Read the model definition and answer for the solid it produces. Units are mm, in the model's axes. A direction names the side the tool comes from. Give positions to 0.01 mm unless a question says otherwise; leave off trailing zeros. Order: outer loops, then holes, each group sorted by start corner. A loop starts at its lowest first (then second) coordinate and runs counter-clockwise, first axis right, second up. Notation, with made-up numbers: (76, 44.5) - (86, 44.5) arc R12 cw to (86, 61.5) - close; hole circle Ø6 at (11, 42). An arc over 180 degrees is marked (long way). One line per item, written item: value. Start each with the question number.
```python
from build123d import *

# Parameters (mm, degrees)
BOSS_EXTRU_1_DEPTH      = 3
ESQUISSE2_R             = 1.5
ENL_V_MAT_EXTRU_2_DEPTH = 3
ESQUISSE3_R             = 6
ESQUISSE3_R_2           = 1.5
ENL_V_MAT_EXTRU_3_DEPTH = 10


with BuildPart() as part:
    # Esquisse1 → Boss.-Extru.1 (new body)
    with BuildSketch(Plane.XY):
        Polygon((-50, -75), (50, -75), (50, -65), (60, -65), (60, 75), (-60, 75), (-60, -65), (-50, -65), align=None)
        with BuildLine():
            ThreePointArc((-41.5, 22), (-43, 20.5), (-44.5, 22))
            Line((-44.5, 22), (-44.5, 37))
            ThreePointArc((-44.5, 37), (-43, 38.5), (-41.5, 37))
            Line((-41.5, 37), (-41.5, 22))
        make_face(mode=Mode.SUBTRACT)
        with BuildLine():
            Line((-10.5, 37), (-10.5, 22))
            ThreePointArc((-10.5, 22), (-12, 20.5), (-13.5, 22))
            Line((-13.5, 22), (-13.5, 37))
            ThreePointArc((-13.5, 37), (-12, 38.5), (-10.5, 37))
        make_face(mode=Mode.SUBTRACT)
        with BuildLine():
            ThreePointArc((-41.5, 53), (-43, 51.5), (-44.5, 53))
            Line((-44.5, 53), (-44.5, 68))
            ThreePointArc((-44.5, 68), (-43, 69.5), (-41.5, 68))
            Line((-41.5, 68), (-41.5, 53))
        make_face(mode=Mode.SUBTRACT)
        with BuildLine():
            ThreePointArc((-16.25, 37.5), (-27.5, 26.25), (-38.75, 37.5))
            Line((-38.75, 37.5), (-38.75, 52.5))
            ThreePointArc((-38.75, 52.5), (-27.5, 63.75), (-16.25, 52.5))
            Line((-16.25, 52.5), (-16.25, 37.5))
        make_face(mode=Mode.SUBTRACT)
        with BuildLine():
            Line((-10.5, 68), (-10.5, 53))
            ThreePointArc((-10.5, 53), (-12, 51.5), (-13.5, 53))
            Line((-13.5, 53), (-13.5, 68))
            ThreePointArc((-13.5, 68), (-12, 69.5), (-10.5, 68))
        make_face(mode=Mode.SUBTRACT)
    extrude(amount=BOSS_EXTRU_1_DEPTH)

    # Esquisse2 → Enlèv. mat.-Extru.2 (cut)
    with BuildSketch(Plane.XY.offset(3)):
        with Locations((45, -70)):
            Circle(ESQUISSE2_R)
        with Locations((-55, -60)):
            Circle(ESQUISSE2_R)
        with Locations((-55, 5)):
            Circle(ESQUISSE2_R)
        with Locations((-55, 70)):
            Circle(ESQUISSE2_R)
        with Locations((22.5, -70)):
            Circle(ESQUISSE2_R)
        with Locations((0, -70)):
            Circle(ESQUISSE2_R)
        with Locations((-22.5, -70)):
            Circle(ESQUISSE2_R)
        with Locations((-45, -70)):
            Circle(ESQUISSE2_R)
        with Locations(Location((55, -60, 0), (0, 0, 180))):
            Circle(ESQUISSE2_R)
        with Locations(Location((55, 5, 0), (0, 0, 180))):
            Circle(ESQUISSE2_R)
        with Locations(Location((55, 70, 0), (0, 0, 180))):
            Circle(ESQUISSE2_R)
    extrude(amount=-ENL_V_MAT_EXTRU_2_DEPTH, mode=Mode.SUBTRACT)

    # Esquisse3 → Enlèv. mat.-Extru.3 (cut)
    with BuildSketch(Plane.XY.offset(3)):
        with Locations((0, -40)):
            Circle(ESQUISSE3_R)
        with Locations((-7.5, -32.5)):
            Circle(ESQUISSE3_R_2)
        with Locations((7.5, -32.5)):
            Circle(ESQUISSE3_R_2)
        with Locations((7.5, -47.5)):
            Circle(ESQUISSE3_R_2)
        with Locations((-7.5, -47.5)):
            Circle(ESQUISSE3_R_2)
    extrude(amount=-ENL_V_MAT_EXTRU_3_DEPTH, mode=Mode.SUBTRACT)


solid = part.part
```
1) Section A-A on y = 28.5 is taken. Write down the section's boundary in (x, z), plus the area to 4 significant figures.
2) Find the intervals of material crossed by probe 1 along X at (y, z) = (70, 2.1); probe 2 along Y at (x, z) = (-45, 0.8); probe 3 along X at (y, z) = (-39.5, 2.7), in increasing order. Write a range as from..to.
3) Section B-B on x = -30.5 is taken. Write down the section's boundary in (y, z), plus the area to 3 significant figures.
4) For faces 1 (the flat face through (-1, 1, 0)), 2 (the flat face through (-44.5, 60, 1)), determine the directions among +Z, -Z, +X, -X, +Y, -Y from which every point of the face is accessible in a straight line to the end or side of a thin tool.
5) Section C-C on z = 2.4 is taken. Give the number of separate pieces and of enclosed holes in the cut face, plus the area to 3 significant figures.
6) Each of these flat-tipped pins is pushed along its axis until it touches: pin 1 (2.5 mm diameter, centred on x = 7.5, y = -32.5, fed in from -Z); pin 2 (0.9 mm diameter, centred on y = -71.5, z = 1.5, fed in from +X). Where does it stop, or does it pass through?
7) The mould has two halves that part along X. Classify faces 3 (the cylindrical face through (-8.7, -33.4, 1.5)), 4 (the flat face through (-50, -70, 1)), 5 (the flat face through (-55, -65, 1)): +X half, -X half, draft (parallel to the pull), parting line (faces both ways), or undercut.
Solved:
1. outline: (-60, 0) - (-44.5, 0) - (-44.5, 3) - (-60, 3) - close; (-41.5, 0) - (-34.25, 0) - (-34.25, 3) - (-41.5, 3) - close; (-20.75, 0) - (-13.5, 0) - (-13.5, 3) - (-20.75, 3) - close; (-10.5, 0) - (60, 0) - (60, 3) - (-10.5, 3) - close
1. area: 301.5 mm2
2. probe 1: x = -60..-56.5, -53.5..53.5, 56.5..60
2. probe 2: y = -75..-71.5, -68.5..75
2. probe 3: x = -60..-5.98, 5.98..60
3. outline: (-75, 0) - (26.66, 0) - (26.66, 3) - (-75, 3) - close; (63.34, 0) - (75, 0) - (75, 3) - (63.34, 3) - close
3. area: 340 mm2
4. face 1: -Z, +X, -X, +Y, -Y
4. face 2: +Z, -Z
5. separate pieces: 1
5. enclosed holes: 21
5. area: 16,600 mm2
6. pin 1: passes through
6. pin 2: stops at x = 50
7. face 3: undercut
7. face 4: -X half
7. face 5: draft
